from build123d import *

# Parameters (mm, degrees)
CROQUIS2_W              = 63.5
CROQUIS2_H              = 50.8
SALIENTE_EXTRUIR1_DEPTH = 254
CROQUIS5_R              = 3.175
CORTAR_EXTRUIR3_DEPTH   = 50.8
CROQUIS10_R             = 4.75
CORTAR_EXTRUIR5_DEPTH   = 8
CORTAR_EXTRUIR6_DEPTH   = 254
CROQUIS12_R             = 4.75
CORTAR_EXTRUIR7_DEPTH   = 8


with BuildPart() as part:
    # Croquis2 → Saliente-Extruir1 (new body)
    with BuildSketch(Plane.XY):
        with Locations((31.75, 25.4)):
            Rectangle(CROQUIS2_W, CROQUIS2_H)
    extrude(amount=-SALIENTE_EXTRUIR1_DEPTH)

    # Croquis5 → Cortar-Extruir3 (cut)
    with BuildSketch(Plane(origin=(0, 50.8, 0), x_dir=(1, 0, 0), z_dir=(0, 1, 0))):
        with Locations((57.82, 5.675)):
            Circle(CROQUIS5_R)
        with Locations((5.68, 5.675)):
            Circle(CROQUIS5_R)
        with Locations((5.68, 248.325)):
            Circle(CROQUIS5_R)
        with Locations((57.82, 248.325)):
            Circle(CROQUIS5_R)
    extrude(amount=-CORTAR_EXTRUIR3_DEPTH, mode=Mode.SUBTRACT)

    # Croquis10 → Cortar-Extruir5 (cut)
    with BuildSketch(Plane(origin=(0, 50.8, 0), x_dir=(1, 0, 0), z_dir=(0, 1, 0))):
        with Locations((57.82, 5.675)):
            Circle(CROQUIS10_R)
        with Locations((5.68, 5.675)):
            Circle(CROQUIS10_R)
    extrude(amount=-CORTAR_EXTRUIR5_DEPTH, mode=Mode.SUBTRACT)

    # Croquis11 → Cortar-Extruir6 (cut)
    with BuildSketch(Plane.XY):
        Polygon((31.75, 31.75), (50.8, 50.8), (12.7, 50.8), align=None)
    extrude(amount=-CORTAR_EXTRUIR6_DEPTH, mode=Mode.SUBTRACT)

    # Croquis12 → Cortar-Extruir7 (cut)
    with BuildSketch(Plane(origin=(0, 50.8, 0), x_dir=(1, 0, 0), z_dir=(0, 1, 0))):
        with Locations((57.82, 248.325)):
            Circle(CROQUIS12_R)
        with Locations((5.68, 248.325)):
            Circle(CROQUIS12_R)
    extrude(amount=-CORTAR_EXTRUIR7_DEPTH, mode=Mode.SUBTRACT)


solid = part.part
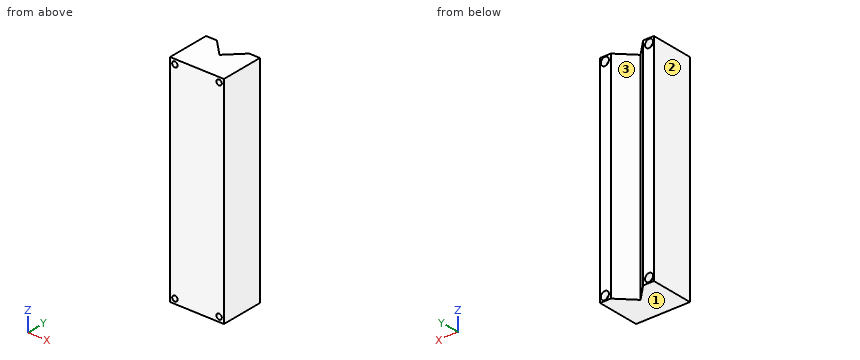
Source: CAD feature listing. Evaluate the final solid. Frame: model axes, mm. Face numbers are marked on the shaded views. Coordinates: 2 decimals unless noted, no trailing zeros. Order: outer loops, then holes, each group sorted by start corner. A loop starts at its lowest first (then second) coordinate and runs counter-clockwise, first axis right, second up. Notation, with made-up numbers: M 72,-16 L 108,-16 A30 cw 108,10 Z; hole C 36.25,14.25 d5. An arc over 180 degrees is marked long. Write each question's results on one line, items separated by ' | '. Start each with the question number.
1. Section B-B, the plane z = -196. Return the cut outline in (x, y), then the cut area to 3 significant figures.
2. Section A-A, the plane x = 5.68. Return the cut outline in (y, z) (3 decimals), then the cut area to 3 significant figures.
3. Draft query along X for the marked faces 1, 2 and 3. Return one class per face: +X half, -X half, draft (parallel to the pull), parting line (faces both ways), or undercut.
4. Section D-D, the plane x = 57. Return the cut outline in (y, z), then the cut area to 3 significant figures.
5. Pin query (flat end, axial travel): pin 1 (8.5 mm diameter, centred on x = 5.68, z = -248.325, fed in from +Y); pin 2 (2 mm diameter, centred on x = 23.5, z = -207, fed in from +Y); pin 3 (10 mm diameter, centred on x = 38.5, z = -82, fed in from -Y); pin 4 (4 mm diameter, centred on x = 57.82, z = -5.675, fed in from -Y). Return the tip coordinate at first contact, or that it passes through.
6. Material intervals for L1, parallel to Z at x = 57.82, y = 16.5; L2, parallel to Z at x = 60.5, y = 17; L3, parallel to X at y = 41.5, z = -39, sorted ascending.
7. Section C-C, the plane x = 17. Return the cut outline in (y, z), then the cut area to 3 significant figures.
Solution:
1) outline: M 0,0 L 63.5,0 L 63.5,50.8 L 50.8,50.8 L 31.75,31.75 L 12.7,50.8 L 0,50.8 Z | area: 2,860 mm²
2) outline: M 0,-254 L 50.8,-254 L 50.8,-253.075 L 42.8,-253.075 L 42.8,-251.5 L 0,-251.5 Z; M 0,-245.15 L 42.8,-245.15 L 42.8,-243.575 L 50.8,-243.575 L 50.8,-10.425 L 42.8,-10.425 L 42.8,-8.85 L 0,-8.85 Z; M 0,-2.5 L 42.8,-2.5 L 42.8,-0.925 L 50.8,-0.925 L 50.8,0 L 0,0 Z | area: 12,200 mm²
3) face 1: draft | face 2: -X half | face 3: undercut
4) outline: M 0,-254 L 50.8,-254 L 50.8,-253 L 42.8,-253 L 42.8,-251.39 L 0,-251.39 Z; M 0,-245.26 L 42.8,-245.26 L 42.8,-243.65 L 50.8,-243.65 L 50.8,-10.35 L 42.8,-10.35 L 42.8,-8.74 L 0,-8.74 Z; M 0,-2.61 L 42.8,-2.61 L 42.8,-1 L 50.8,-1 L 50.8,0 L 0,0 Z | area: 12,200 mm²
5) pin 1: y = 42.8 | pin 2: y = 41 | pin 3: y = 0 | pin 4: through
6) L1: -254 to -251.5, -245.15 to -8.85, -2.5 to 0 | L2: -254 to -250.03, -246.62 to -7.38, -3.97 to 0 | L3: 0 to 22, 41.5 to 63.5
7) outline: M 0,-254 L 46.5,-254 L 46.5,0 L 0,0 Z | area: 11,800 mm²
